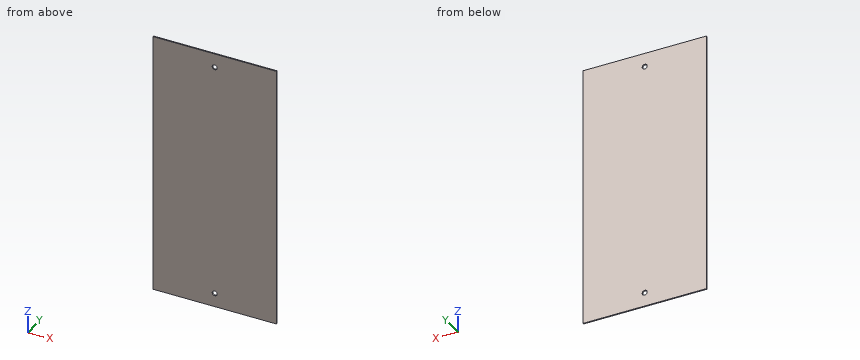
```python
from build123d import *

# Parameters (mm, degrees)
ESBO_O1_W                   = 220
ESBO_O1_H                   = 2
RESSALTO_EXTRUS_O1_DEPTH    = 475
FURO_COM_FOLGA_DE_M81_D     = 9
FURO_COM_FOLGA_DE_M81_DEPTH = 10
FURO_COM_FOLGA_DE_M81_TIP   = 2.703872786


with BuildPart() as part:
    # Esboço1 → Ressalto-extrusão1 (new body)
    with BuildSketch(Plane.XY):
        with Locations((110, 1)):
            Rectangle(ESBO_O1_W, ESBO_O1_H)
    extrude(amount=RESSALTO_EXTRUS_O1_DEPTH)

    # Furo com folga de M81
    with Locations(Plane(origin=(110, 2, 25), x_dir=(0, 0, 1), z_dir=(0, 1, 0))):
        with Locations((0, 0), (425, 0)):
            Hole(FURO_COM_FOLGA_DE_M81_D / 2, depth=FURO_COM_FOLGA_DE_M81_DEPTH)
            with Locations((0, 0, -(FURO_COM_FOLGA_DE_M81_DEPTH + FURO_COM_FOLGA_DE_M81_TIP / 2))):  # 118° drill point
                Cone(0, FURO_COM_FOLGA_DE_M81_D / 2, FURO_COM_FOLGA_DE_M81_TIP, mode=Mode.SUBTRACT)


solid = part.part
```
Geometry: final body of the model. Coordinates: model frame, mm. Give positions to 0.01 mm unless a question says otherwise; leave off trailing zeros. Order: outer loops, then holes, each group sorted by start corner. A loop starts at its lowest first (then second) coordinate and runs counter-clockwise, first axis right, second up. Notation, with made-up numbers: M 33.5,46.5 L 44.5,46.5 A34 cw 44.5,85.5 Z; hole C 75.25,75 d11. An arc over 180 degrees is marked long. Answer as CSV lines item,"result". Start each with the question number.
1) Line query: line 1 (X direction, y = 0.6, z = 450); line 2 (X direction, y = 1.85, z = 24). Output: solid intervals per line, ascending. Write a range as from..to.
2) First-contact query: P1, Ø5.5, axis at x = 110, z = 450, coming from the -Y side; P2, Ø11.5, axis at x = 110, z = 25, coming from the -Y side. Flat tips, straight axial feed; report the tip coordinate or a pass-through.
3) Cut plane A-A (x = 110). Output: boundary loops of the cut face in (y, z), then the cut area to 3 significant figures.
4) Cut plane B-B (z = 450). Output: boundary loops of the cut face in (x, y).
Findings below:
1,line 1,"x = 0..105.5, 114.5..220"
1,line 2,"x = 0..105.61, 114.39..220"
2,P1,"passes through"
2,P2,"stops at y = 0"
3,outline,"M 0,0 L 2,0 L 2,20.5 L 0,20.5 Z; M 0,29.5 L 2,29.5 L 2,445.5 L 0,445.5 Z; M 0,454.5 L 2,454.5 L 2,475 L 0,475 Z"
3,area,"914 mm²"
4,outline,"M 0,0 L 105.5,0 L 105.5,2 L 0,2 Z; M 114.5,0 L 220,0 L 220,2 L 114.5,2 Z"
